from build123d import *

# Parameters (mm, degrees)
SKETCH1_R           = 65
BOSS_EXTRUDE1_DEPTH = 3
SKETCH2_R           = 3
CUT_EXTRUDE1_DEPTH  = 4
CIRPATTERN1_COUNT   = 4
SKETCH3_R           = 40
CUT_EXTRUDE2_DEPTH  = 4


with BuildPart() as part:
    # Sketch1 → Boss-Extrude1 (new body)
    with BuildSketch(Plane(origin=(0, 0, 0), x_dir=(1, 0, 0), z_dir=(0, 1, 0))):
        Circle(SKETCH1_R)
    extrude(amount=BOSS_EXTRUDE1_DEPTH)

    # Sketch2 → Cut-Extrude1 (cut, through all)
    with BuildSketch(Plane(origin=(0, 3, 0), x_dir=(1, 0, 0), z_dir=(0, 1, 0))):
        with Locations((0, 55)):
            Circle(SKETCH2_R)
    cut_extrude1 = extrude(amount=-CUT_EXTRUDE1_DEPTH, mode=Mode.SUBTRACT)

    # CirPattern1: Cut-Extrude1 ×4 about axis
    cirpattern1_axis = Axis((0, 0, 0), (0, 1, 0))
    for i in range(1, CIRPATTERN1_COUNT):
        add(cut_extrude1.rotate(cirpattern1_axis, i * 360 / CIRPATTERN1_COUNT), mode=Mode.SUBTRACT)

    # Sketch3 → Cut-Extrude2 (cut, through all)
    with BuildSketch(Plane(origin=(0, 3, 0), x_dir=(1, 0, 0), z_dir=(0, 1, 0))):
        Circle(SKETCH3_R)
    extrude(amount=-CUT_EXTRUDE2_DEPTH, mode=Mode.SUBTRACT)


solid = part.part
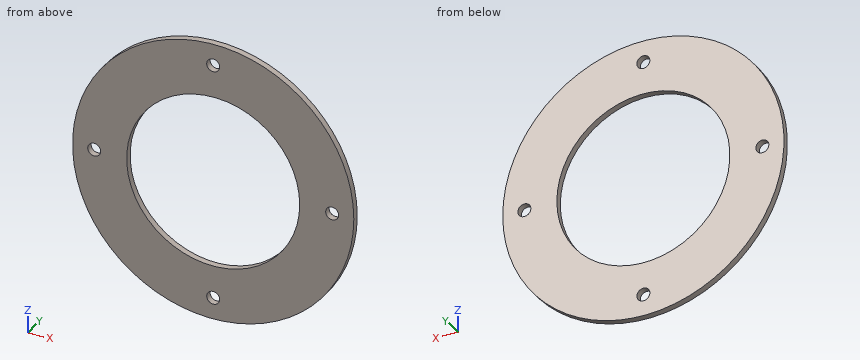
The model under review builds one solid part; all positions refer to its coordinate system, in mm. Coordinates: 2 decimals unless noted, no trailing zeros. Write each loop counter-clockwise with the first axis right and the second up, starting at its lowest first coordinate (ties: lowest second). Pieces come first, ordered by that corner, then holes. Notation, with made-up numbers: (44, -29) - (87, -29) arc R30 ccw to (87, 6) - close; hole circle Ø11 at (61.5, 4). An arc over 180 degrees is marked (long way). Answer as a JSON object with one key per item and string values. Group by question number.
1. Add section A-A (z = 0). Give the boundary of the cut face in (x, y), plus the area to 3 significant figures.
2. Add section C-C (x = 0). Give the boundary of the cut face in (y, z), plus the area to 3 significant figures.
3. Add section D-D (z = 24). Give the boundary of the cut face in (x, y), plus the area to 3 significant figures.
4. To check wall thickness, follow probe 1 along Z at (x, y) = (0, 1.5); probe 2 along Z at (x, y) = (-1, 1.25); probe 3 along X at (y, z) = (0.5, -35). State the ranges of each line that lie inside material, in increasing order.
5. Add section B-B (y = 2.15). Give the boundary of the cut face in (x, z).
6. Clearance check with flat-ended pins moving along their axes: pin 1 Ø1.5 at (x, y) = (4, 2.5) entering from -Z; pin 2 Ø5 at (x, z) = (-55, 0) entering from +Y. State where each tip first meets the part, or that it passes through.
Findings:
{
 "1": {"outline": "(-65, 0) - (-58, 0) - (-58, 3) - (-65, 3) - close; (-52, 0) - (-40, 0) - (-40, 3) - (-52, 3) - close; (40, 0) - (52, 0) - (52, 3) - (40, 3) - close; (58, 0) - (65, 0) - (65, 3) - (58, 3) - close", "area": "114 mm²"},
 "2": {"outline": "(0, -65) - (3, -65) - (3, -58) - (0, -58) - close; (0, -52) - (3, -52) - (3, -40) - (0, -40) - close; (0, 40) - (3, 40) - (3, 52) - (0, 52) - close; (0, 58) - (3, 58) - (3, 65) - (0, 65) - close", "area": "114 mm²"},
 "3": {"outline": "(-60.41, 0) - (-32, 0) - (-32, 3) - (-60.41, 3) - close; (32, 0) - (60.41, 0) - (60.41, 3) - (32, 3) - close", "area": "170 mm²"},
 "4": {"probe 1": "-65 to -58, -52 to -40, 40 to 52, 58 to 65", "probe 2": "-64.99 to -57.83, -52.17 to -39.99, 39.99 to 52.17, 57.83 to 64.99", "probe 3": "-54.77 to -19.36, 19.36 to 54.77"},
 "5": {"outline": "circle Ø130 at (0, 0); hole circle Ø6 at (-55, 0); hole circle Ø80 at (0, 0); hole circle Ø6 at (0, -55); hole circle Ø6 at (0, 55); hole circle Ø6 at (55, 0)"},
 "6": {"pin 1": "z = -64.92", "pin 2": "through"}
}
